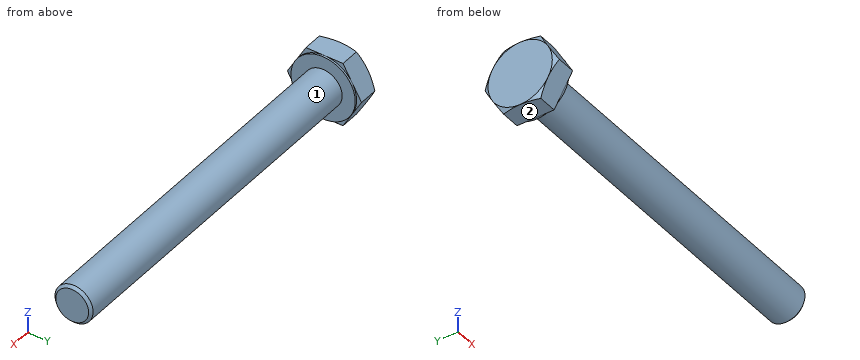
```python
from build123d import *

# Parameters (mm, degrees)
BASEHEAD_DEPTH = 10
SKETCH4_W      = 0.8
SKETCH4_H      = 12.088457268


# Read off the part's stored shape, not the designer's step: HeadChamfer
with BuildPart() as part:
    # Sketch1 → BaseHead (new body)
    with BuildSketch(Plane(origin=(0, 0, 0), x_dir=(0, 0, -1), z_dir=(1, 0, 0))):
        Polygon((13.5, 7.794228634), (13.5, -7.794228634), (0, -15.588457268), (-13.5, -7.794228634), (-13.5, 7.794228634), (0, 15.588457268), align=None)
    extrude(amount=BASEHEAD_DEPTH)

    # HeadChamfer outline → HeadChamfer (revolve, cut)
    with BuildSketch(Plane.YX):
        Polygon((15.58845727, 1.205771367), (13.499999851, -8.6e-08), (15.58845727, -8.6e-08), align=None)
    revolve(axis=Axis((0, 0, 0), (1, 0, 0)), mode=Mode.SUBTRACT)

    # HeadChamfer 2 outline → HeadChamfer 2 (revolve)
    with BuildSketch(Plane.YX):
        Polygon((8, 10), (8, 158.8985), (6.8985, 160), (0, 160), (0, 10), align=None)
    revolve(axis=Axis((0, 0, 0), (1, 0, 0)))

    # Sketch4 → BearingFace (revolve, cut)
    with BuildSketch(Plane.XY, mode=Mode.PRIVATE) as bearingface_sk:
        with Locations((9.6, 19.544228634)):
            Rectangle(SKETCH4_W, SKETCH4_H)
    revolve(bearingface_sk.sketch.rotate(Axis((0, 0, 0), (1, 0, 0)), 90), axis=Axis((0, 0, 0), (1, 0, 0)), mode=Mode.SUBTRACT)


solid = part.part
```
Part model, mm, in its own coordinate system. Face numbers are marked on the shaded views. A direction names the side the tool comes from. Round coordinates to 2 decimals unless told otherwise and drop trailing zeros. Loops run counter-clockwise (first coordinate to the right, second up) from the corner with the lowest first, then second, coordinate; pieces in that order, holes last. Notation, with made-up numbers: (1, 85.25) -> (59, 85.25) arc R9 ccw to (59, 91.25) -> close; hole circle Ø2 at (-30.5, -14). An arc over 180 degrees is marked (long way). Use a Markdown table: item, result.
1) Tool access for the marked faces 1 and 2: list every direction of +Z, -Z, +X, -X, +Y, -Y with a clear straight run to the whole face (end or side of a thin tool).
The answers:
| item | result |
|---|---|
| face 1 | +X |
| face 2 | -Z, +X, -X, +Y, -Y |
2) Probe line 1 (Z direction, x = 23, y = -0.5); line 2 (X direction, y = 1.5, z = -8); line 3 (Y direction, x = 106, z = -4). List the from-to ranges inside material, lowest first. Write a range as [from, to].
The answers:
| item | result |
|---|---|
| line 1 | z = [-7.98, 7.98] |
| line 2 | x = [0, 10] |
| line 3 | y = [-6.93, 6.93] |
3) Drop flat-ended pins along their axis: pin 1 Ø2 at (x, y) = (19, -3) entering from +Z; pin 2 Ø3.5 at (y, z) = (5, -11.5) entering from +X; pin 3 Ø12 at (x, y) = (22, -2) entering from -Z; pin 4 Ø8 at (y, z) = (-8, 4) entering from +X. Give the stop position or say it passes through.
The answers:
| item | result |
|---|---|
| pin 1 | stops at z = 7.75 |
| pin 2 | stops at x = 10 |
| pin 3 | stops at z = -8 |
| pin 4 | stops at x = 160 |
4) Cut at A-A, the plane x = 31.5. List the corners of the cut face in (y, z), and give its area (3 significant figures).
The answers:
| item | result |
|---|---|
| outline | circle Ø16 at (0, 0) |
| area | 201 mm2 |
